from build123d import *

# Parameters (mm, degrees)
CROQUIS1_W              = 38.1
CROQUIS1_H              = 850.5
SALIENTE_EXTRUIR1_DEPTH = 6.31
CROQUIS2_W              = 38.1
CROQUIS2_H              = 6.31
SALIENTE_EXTRUIR2_DEPTH = 70
CROQUIS3_W              = 38.1
CROQUIS3_H              = 6.31
SALIENTE_EXTRUIR3_DEPTH = 578
CROQUIS4_R              = 6.935856655
CORTAR_EXTRUIR1_DEPTH   = 7
CROQUIS5_W              = 38.1
CROQUIS5_H              = 687.72607772
CORTAR_EXTRUIR2_DEPTH   = 10
CROQUIS6_W              = 38.1
CROQUIS6_H              = 6.31
CROQUIS8_W              = 368.89
CROQUIS8_H              = 6.31
CORTAR_EXTRUIR3_DEPTH   = 147
CROQUIS9_R              = 6.35
CORTAR_EXTRUIR4_DEPTH   = 6.31
CROQUIS10_W             = 38.1
CROQUIS10_H             = 6.31


with BuildPart() as part:
    # Croquis1 → Saliente-Extruir1 (new body)
    with BuildSketch(Plane.XY):
        Rectangle(CROQUIS1_W, CROQUIS1_H)
    extrude(amount=SALIENTE_EXTRUIR1_DEPTH)

    # Croquis2 → Saliente-Extruir2 (add)
    with BuildSketch(Plane.XY.offset(6.31)):
        with Locations((0, -422.095)):
            Rectangle(CROQUIS2_W, CROQUIS2_H)
    extrude(amount=SALIENTE_EXTRUIR2_DEPTH)

    # Croquis3 → Saliente-Extruir3 (add)
    with BuildSketch(Plane.XY.offset(6.31)):
        with Locations((0, -265.63107772)):
            Rectangle(CROQUIS3_W, CROQUIS3_H)
    extrude(amount=-SALIENTE_EXTRUIR3_DEPTH)

    # Croquis4 → Cortar-Extruir1 (cut)
    with BuildSketch(Plane(origin=(0, -262.47607772, 0), x_dir=(1, 0, 0), z_dir=(0, 1, 0))):
        with Locations(Location((0, 536.981534281, 0), (0, 0, 270))):
            Circle(CROQUIS4_R)
    extrude(amount=-CORTAR_EXTRUIR1_DEPTH, mode=Mode.SUBTRACT)

    # Croquis5 → Cortar-Extruir2 (cut)
    with BuildSketch(Plane(origin=(0, 0, 0), x_dir=(-1, 0, 0), z_dir=(0, 0, -1))):
        with Locations((0, 81.38696114)):
            Rectangle(CROQUIS5_W, CROQUIS5_H)
    extrude(amount=-CORTAR_EXTRUIR2_DEPTH, mode=Mode.SUBTRACT)

    # Barrer1: sweep along a curve in space
    with BuildLine() as barrer1_path:
        Line((0, -262.47607772, -199.645), (0, 386.85392228, -199.645))
        Line((0, 386.85392228, -199.645), (0, 386.85392228, 127.905))
    # Croquis6 → Barrer1 (sweep)
    with BuildSketch(Plane(origin=(0, -262.47607772, 0), x_dir=(1, 0, 0), z_dir=(0, 1, 0))):
        with Locations((0, 199.645)):
            Rectangle(CROQUIS6_W, CROQUIS6_H)
    sweep(path=barrer1_path.line, transition=Transition.RIGHT)

    # Croquis8 → Cortar-Extruir3 (cut)
    with BuildSketch(Plane(origin=(19.05, 0, 0), x_dir=(0, 0, -1), z_dir=(1, 0, 0))):
        Polygon((196.49, -262.47607772), (196.49, -268.78607772), (196.49, -444.307673596), (-90.834600665, -444.307673596), (-90.834600665, -262.47607772), align=None)
        with Locations((387.245, -265.63107772)):
            Rectangle(CROQUIS8_W, CROQUIS8_H)
    extrude(amount=-CORTAR_EXTRUIR3_DEPTH, mode=Mode.SUBTRACT)

    # Croquis9 → Cortar-Extruir4 (cut)
    with BuildSketch(Plane(origin=(0, 390.00892228, 0), x_dir=(1, 0, 0), z_dir=(0, 1, 0))):
        with Locations(Location((0, -84.010000001, 0), (0, 0, 180))):
            Circle(CROQUIS9_R)
        with Locations(Location((0, -116.010000001, 0), (0, 0, 180))):
            Circle(CROQUIS9_R)
    extrude(amount=-CORTAR_EXTRUIR4_DEPTH, mode=Mode.SUBTRACT)

    # Barrer2: sweep along a curve in space
    with BuildLine() as barrer2_path:
        Line((0, -268.78607772, -199.645), (0, -278.78607772, -199.645))
        Line((0, -278.78607772, -199.645), (0, -278.78607772, -101.215))
        Line((0, -278.78607772, -101.215), (0, -342.02607772, -101.215))
    # Croquis10 → Barrer2 (sweep)
    with BuildSketch(Plane.XZ.offset(268.78607772)):
        with Locations((0, -199.645)):
            Rectangle(CROQUIS10_W, CROQUIS10_H)
    sweep(path=barrer2_path.line, transition=Transition.RIGHT)


solid = part.part
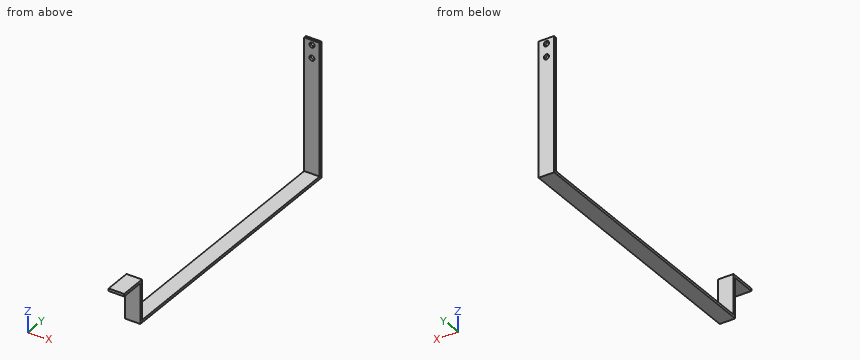
Input: part model. Units: mm. Frame: model coordinates. Give positions to 0.01 mm unless a question says otherwise; leave off trailing zeros. Order: outer loops, then holes, each group sorted by start corner. A loop starts at its lowest first (then second) coordinate and runs counter-clockwise, first axis right, second up.
Q1. Section B-B on x = 0. Output: boundary loops of the cut face in (y, z) (3 decimals).
Checked values:
outline: (-342.026, -104.37) - (-281.941, -104.37) - (-281.941, -202.8) - (390.009, -202.8) - (390.009, 77.66) - (383.699, 77.66) - (383.699, -196.49) - (-275.631, -196.49) - (-275.631, -98.06) - (-342.026, -98.06) - close; (383.699, 90.36) - (390.009, 90.36) - (390.009, 109.66) - (383.699, 109.66) - close; (383.699, 122.36) - (390.009, 122.36) - (390.009, 127.905) - (383.699, 127.905) - close
Q2. Section C-C on z = 68. Output: boundary loops of the cut face in (x, y), and give its area (3 significant figures).
Checked values:
outline: (-19.05, 383.7) - (19.05, 383.7) - (19.05, 390.01) - (-19.05, 390.01) - close
area: 240 mm2
Q3. Contact query for flat-ended pins moving along their axis: pin 1 Ø4 at (x, z) = (5.5, 66.5) entering from -Y; pin 2 Ø1 at (x, y) = (6.5, -10.5) entering from +Z; pin 3 Ø11.5 at (x, y) = (9.5, -316.5) entering from +Z. Output: stop coordinate, or through.
Checked values:
pin 1: stops at y = 383.7
pin 2: stops at z = -196.49
pin 3: stops at z = -98.06
Q4. Section D-D on y = -32. Output: boundary loops of the cut face in (x, z), and give its area (3 significant figures).
Checked values:
outline: (-19.05, -202.8) - (19.05, -202.8) - (19.05, -196.49) - (-19.05, -196.49) - close
area: 240 mm2
Q5. Section A-A on z = -165. Output: boundary loops of the cut face in (x, y).
Checked values:
outline: (-19.05, -281.94) - (19.05, -281.94) - (19.05, -275.63) - (-19.05, -275.63) - close; (-19.05, 383.7) - (19.05, 383.7) - (19.05, 390.01) - (-19.05, 390.01) - close
Q6. Ray query, probe 1 along Z at (x, y) = (0, 387) (3 decimals); probe 2 along Y at (x, z) = (-12, -149); probe 3 along X at (y, z) = (386, 116). Return the intervals inside material, ascending.
Checked values:
probe 1: z = -202.8 to 77.66, 90.36 to 109.66, 122.36 to 127.905
probe 2: y = -281.94 to -275.63, 383.7 to 390.01
probe 3: x = -19.05 to -6.35, 6.35 to 19.05
